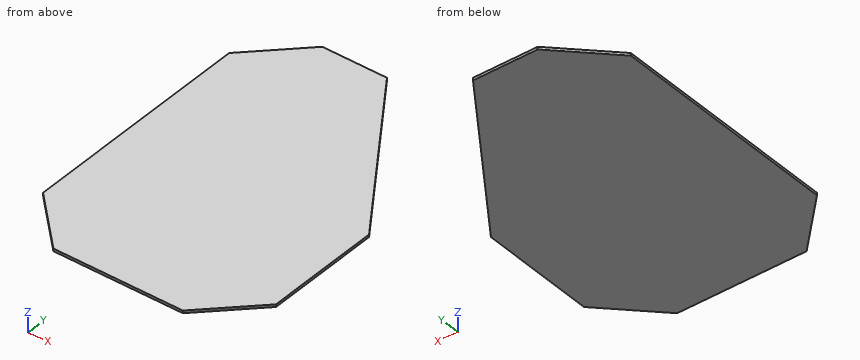
from build123d import *

# Parameters (mm, degrees)
F1_DEPTH = 1
F2_SIZE  = 20
F3_SIZE  = 20
F4_SIZE  = 20


with BuildPart() as f1:
    # F0 (on Top) → F1 (new body)
    with BuildSketch(Plane.XY):
        Polygon((6.802157, 69.381405), (-38.197843, 69.381405), (-38.197843, -60.618595), (51.802157, -60.618595), (51.802157, 4.381405), align=None)
    extrude(amount=F1_DEPTH)

    # F2
    f2_edges = [f1.edges().sort_by_distance(p)[0] for p in [
        (51.802157, -60.618595, 0.5),
    ]]
    chamfer(f2_edges, length=F2_SIZE)

    # F3
    f3_edges = [f1.edges().sort_by_distance(p)[0] for p in [
        (-38.197843, -60.618595, 0.5),
    ]]
    chamfer(f3_edges, length=F3_SIZE)

    # F4
    f4_edges = [f1.edges().sort_by_distance(p)[0] for p in [
        (-38.197843, 69.381405, 0.5),
    ]]
    chamfer(f4_edges, length=F4_SIZE)


solid = f1.part
For this review, take the finished solid that the model builds, in its own axes (mm). Round coordinates to 2 decimals unless told otherwise and drop trailing zeros. Loops run counter-clockwise (first coordinate to the right, second up) from the corner with the lowest first, then second, coordinate; pieces in that order, holes last. Notation, with made-up numbers: (-12.5, 45.5) - (30.5, 45.5) arc R22 ccw to (30.5, 55.5) - close; hole circle Ø5 at (88.5, -15.75). An arc over 180 degrees is marked (long way). One line per question, with ' | ' between items.
Q1. Take a section at B-B (x = 17). Give the boundary of the cut face in (y, z).
Taken from the geometry:
outline: (-60.62, 0) - (54.65, 0) - (54.65, 1) - (-60.62, 1) - close
Q2. Take a section at A-A (z = 0.7). Give the boundary of the cut face in (x, y).
Taken from the geometry:
outline: (-38.2, -40.62) - (-18.2, -60.62) - (31.8, -60.62) - (51.8, -40.62) - (51.8, 4.38) - (6.8, 69.38) - (-18.2, 69.38) - (-38.2, 49.38) - close
Q3. For line 1 along Y through (x, z) = (44, 0.6); line 2 along Y through (x, z) = (35, 0.85); line 3 along X through (y, z) = (31, 0.7), list the stretches that pass through material, from the lowest coordinate up. Write a range as [from, to].
Taken from the geometry:
line 1: y = [-48.42, 15.65] | line 2: y = [-57.42, 28.65] | line 3: x = [-38.2, 33.37]
Q4. Take a section at C-C (y = 28). Give the boundary of the cut face in (x, z), and give its area (3 significant figures).
Taken from the geometry:
outline: (-38.2, 0) - (35.45, 0) - (35.45, 1) - (-38.2, 1) - close | area: 73.6 mm²
